```python
from build123d import *

# Parameters (mm, degrees)
SKETCH1_W            = 156.5
SKETCH1_H            = 173.5
BOSS_EXTRUDE1_DEPTH  = 5
BOSS_EXTRUDE2_DEPTH  = 17.6
M3_CLEARANCE_HOLE1_D = 3.4
SKETCH6_W            = 50
SKETCH6_H            = 7.5
BOSS_EXTRUDE3_DEPTH  = 20
BOSS_EXTRUDE5_DEPTH  = 10
SKETCH8_W            = 20
SKETCH8_H            = 20
SKETCH8_R            = 1.8
BOSS_EXTRUDE6_DEPTH  = 10
SKETCH9_R            = 1.8
CUT_EXTRUDE1_DEPTH   = 8.5


with BuildPart() as part:
    # Sketch1 → Boss-Extrude1 (new body)
    with BuildSketch(Plane(origin=(0, 0, 0), x_dir=(1, 0, 0), z_dir=(0, 1, 0))):
        Rectangle(SKETCH1_W, SKETCH1_H)
    extrude(amount=-BOSS_EXTRUDE1_DEPTH)

    # Sketch1<2> → Boss-Extrude2 (add)
    with BuildSketch(Plane(origin=(0, 0, 0), x_dir=(1, 0, 0), z_dir=(0, 1, 0))):
        Polygon((-78.25, -7.85), (-68.25, -7.85), (-68.25, 76.75), (-55, 76.75), (-55, 86.75), (-78.25, 86.75), align=None)
        Polygon((68.25, 76.75), (68.25, -7.85), (78.25, -7.85), (78.25, 86.75), (55, 86.75), (55, 76.75), align=None)
        Polygon((68.25, -76.75), (-68.25, -76.75), (-68.25, -62.85), (-78.25, -62.85), (-78.25, -86.75), (78.25, -86.75), (78.25, -62.85), (68.25, -62.85), align=None)
    extrude(amount=BOSS_EXTRUDE2_DEPTH)

    # M3 Clearance Hole1 (through all)
    with Locations(Plane(origin=(0, 0, 0), x_dir=(1, 0, 0), z_dir=(0, 1, 0))):
        with Locations((-63, 69), (-63, -70.35), (63, -70.35), (63, 69)):
            Hole(M3_CLEARANCE_HOLE1_D / 2)

    # Sketch6 → Boss-Extrude3 (add)
    with BuildSketch(Plane.XZ.offset(5)):
        with Locations((-53.25, 83)):
            Rectangle(SKETCH6_W, SKETCH6_H)
        with Locations((-53.25, 58.75)):
            Rectangle(SKETCH6_W, SKETCH6_H)
        with Locations((-53.25, 35.25)):
            Rectangle(SKETCH6_W, SKETCH6_H)
        with Locations((-53.25, 11.75)):
            Rectangle(SKETCH6_W, SKETCH6_H)
        with Locations((53.25, 11.75)):
            Rectangle(SKETCH6_W, SKETCH6_H)
        with Locations((53.25, 35.25)):
            Rectangle(SKETCH6_W, SKETCH6_H)
        with Locations((53.25, 58.75)):
            Rectangle(SKETCH6_W, SKETCH6_H)
        with Locations((53.25, 83)):
            Rectangle(SKETCH6_W, SKETCH6_H)
        with Locations((53.25, -83)):
            Rectangle(SKETCH6_W, SKETCH6_H)
        with Locations((53.25, -58.75)):
            Rectangle(SKETCH6_W, SKETCH6_H)
        with Locations((53.25, -35.25)):
            Rectangle(SKETCH6_W, SKETCH6_H)
        with Locations((53.25, -11.75)):
            Rectangle(SKETCH6_W, SKETCH6_H)
        with Locations((-53.25, -11.75)):
            Rectangle(SKETCH6_W, SKETCH6_H)
        with Locations((-53.25, -35.25)):
            Rectangle(SKETCH6_W, SKETCH6_H)
        with Locations((-53.25, -58.75)):
            Rectangle(SKETCH6_W, SKETCH6_H)
        with Locations((-53.25, -83)):
            Rectangle(SKETCH6_W, SKETCH6_H)
    extrude(amount=BOSS_EXTRUDE3_DEPTH)

    # Sketch7 → Boss-Extrude5 (add)
    with BuildSketch(Plane(origin=(78.25, 0, 0), x_dir=(0, 0, -1), z_dir=(1, 0, 0))):
        Polygon((-86.75, 17.6), (-86.75, 37.6), (-20.098711306, 37.6), (14.542304845, 17.6), align=None)
        Polygon((-76.75, 31.6), (-21.706406461, 31.6), (-7.85, 23.6), (-76.75, 23.6), align=None, mode=Mode.SUBTRACT)
    extrude(amount=-BOSS_EXTRUDE5_DEPTH)

    # Sketch8 → Boss-Extrude6 (add)
    with BuildSketch(Plane.XY.offset(86.75)):
        with Locations((58.25, 27.6)):
            Rectangle(SKETCH8_W, SKETCH8_H)
        with Locations((58.25, 27.6)):
            Circle(SKETCH8_R, mode=Mode.SUBTRACT)
    extrude(amount=-BOSS_EXTRUDE6_DEPTH)

    # Mirror2: part across plane


with BuildPart() as part_1:
    add(part.part)
    add(part.part.mirror(Plane(origin=(0, 0, 0), x_dir=(0, 0, 1), z_dir=(1, 0, 0))))

    # Sketch9 → Cut-Extrude1 (cut, through all)
    with BuildSketch(Plane(origin=(0, 0, 79.25), x_dir=(-1, 0, 0), z_dir=(0, 0, -1))):
        with Locations((-38.25, -15)):
            Circle(SKETCH9_R)
        with Locations((38.25, -15)):
            Circle(SKETCH9_R)
    extrude(amount=-CUT_EXTRUDE1_DEPTH, mode=Mode.SUBTRACT)


solid = part_1.part
```
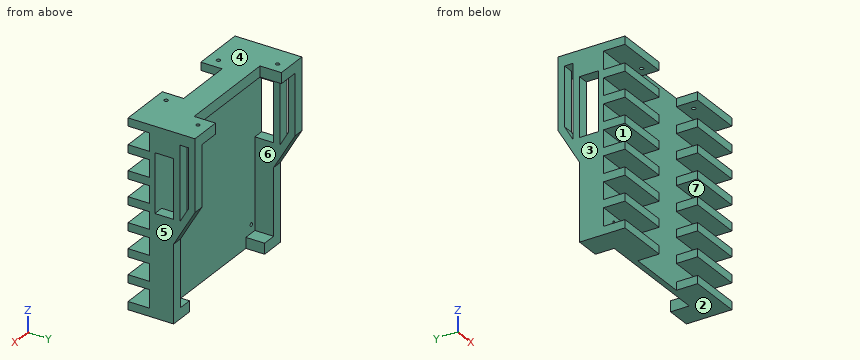
Source: CAD feature listing. Evaluate the final solid. Frame: model axes, mm. Face numbers are marked on the shaded views. A direction names the side the tool comes from. Round coordinates to 2 decimals unless told otherwise and drop trailing zeros. Loops run counter-clockwise (first coordinate to the right, second up) from the corner with the lowest first, then second, coordinate; pieces in that order, holes last.
1. Section query C-C on x = -6. Output: boundary loops of the cut face in (y, z), and give its area (3 significant figures).
2. Section query D-D on z = -5.5. Output: boundary loops of the cut face in (x, y), and give its area (3 significant figures).
3. Mould query, pull axis Z, two halves, no side actions, for the marked faces 1, 2, 3 and 4. Classes: released by +Z, released by -Z, zero draft, split by the parting line, or undercut.
4. Section query B-B on z = 47.5. Output: boundary loops of the cut face in (x, y).
5. Ray query, L1, parallel to X at y = -1.15, z = 70.35; L2, parallel to Z at x = 63, y = -3; L3, parallel to X at y = -16.5, z = 57.5. Return the intervals inside material, ascending.
6. Access query for the marked faces 5, 6 and 7. Directions: +Z, -Z, +X, -X, +Y, -Y. A direction counts if a zero-diameter tool reaches every point of the face in a straight line with its end or side. Return the directions, or none.
7. Contact query for flat-ended pins moving along their axis: pin 1 (3 mm diameter, centred on x = 30, z = 15, fed in from +Y); pin 2 (4 mm diameter, centred on x = 58.25, y = 27.6, fed in from -Z). Output: stop coordinate, or through.
8. Section query A-A on y = 11. Output: boundary loops of the cut face in (x, z).
Answers below:
1. outline: (-5, -86.75) - (0, -86.75) - (0, 76.75) - (17.6, 76.75) - (17.6, 86.75) - (-5, 86.75) - close
1. area: 1,040 mm2
2. outline: (-78.25, -5) - (78.25, -5) - (78.25, 22.82) - (68.25, 22.82) - (68.25, 0) - (-68.25, 0) - (-68.25, 22.82) - (-78.25, 22.82) - close
2. area: 1,240 mm2
3. face 1: undercut
3. face 2: released by -Z
3. face 3: zero draft
3. face 4: released by +Z
4. outline: (-78.25, -5) - (78.25, -5) - (78.25, 0) - (-78.25, 0) - close; (-78.25, 17.6) - (-68.25, 17.6) - (-68.25, 23.6) - (-78.25, 23.6) - close; (-78.25, 31.6) - (-68.25, 31.6) - (-68.25, 37.6) - (-78.25, 37.6) - close; (68.25, 17.6) - (78.25, 17.6) - (78.25, 23.6) - (68.25, 23.6) - close; (68.25, 31.6) - (78.25, 31.6) - (78.25, 37.6) - (68.25, 37.6) - close
5. L1: x = -78.25 to -64.7, -61.3 to 61.3, 64.7 to 78.25
5. L2: z = -86.75 to -70.7, -67.3 to 68.65, 72.05 to 86.75
5. L3: x = -78.25 to -28.25, 28.25 to 78.25
6. face 5: +Z, -Z, +X, +Y, -Y
6. face 6: +Y
6. face 7: +X, -X, -Y
7. pin 1: stops at y = 0
7. pin 2: stops at z = 76.75
8. outline: (-78.25, -86.75) - (-55, -86.75) - (-55, -76.75) - (-68.25, -76.75) - (-68.25, 7.85) - (-78.25, 7.85) - close; (-78.25, 62.85) - (-68.25, 62.85) - (-68.25, 76.75) - (68.25, 76.75) - (68.25, 62.85) - (78.25, 62.85) - (78.25, 86.75) - (-78.25, 86.75) - close; (55, -86.75) - (78.25, -86.75) - (78.25, 7.85) - (68.25, 7.85) - (68.25, -76.75) - (55, -76.75) - close
